```python
from build123d import *

# Parameters (mm, degrees)
SKETCH1_W                          = 70.866
SKETCH1_H                          = 25.4
SKETCH1_W_2                        = 55.372
SKETCH1_H_2                        = 19.9898
BOSS_EXTRUDE1_DEPTH                = 5.08
SKETCH7_W                          = 7.747
SKETCH7_H                          = 25.4
SKETCH7_W_2                        = 7.523824479
BOSS_EXTRUDE2_DEPTH                = 5.08
BOSS_EXTRUDE3_DEPTH                = 25.4
TAP_DRILL_FOR_6_32_TAP1_D          = 2.7051
TAP_DRILL_FOR_6_32_TAP1_DEPTH      = 10.16
TAP_DRILL_FOR_6_32_TAP1_TIP        = 0.81269403
TAP_DRILL_FOR_6_32_TAP2_AT_2_COUNT = 2
TAP_DRILL_FOR_6_32_TAP2_AT_2_PITCH = 12.7


with BuildPart() as part:
    # Sketch1 → Boss-Extrude1 (new body)
    with BuildSketch(Plane(origin=(0, 0, 0), x_dir=(1, 0, 0), z_dir=(0, 1, 0))):
        Rectangle(SKETCH1_W, SKETCH1_H)
        Rectangle(SKETCH1_W_2, SKETCH1_H_2, mode=Mode.SUBTRACT)
    extrude(amount=BOSS_EXTRUDE1_DEPTH)

    # Sketch7 → Boss-Extrude2 (add)
    with BuildSketch(Plane.XZ):
        with Locations((-31.5595, 0)):
            Rectangle(SKETCH7_W, SKETCH7_H)
        with Locations((31.671087761, 0)):
            Rectangle(SKETCH7_W_2, SKETCH7_H)
    extrude(amount=BOSS_EXTRUDE2_DEPTH)

    # Sketch8 → Boss-Extrude3 (add)
    with BuildSketch(Plane.XY.offset(12.7)):
        Polygon((35.433, 5.08), (35.433, -15.24), (39.243, -15.24), (39.243, -5.08), (39.243, 5.08), align=None)
    boss_extrude3 = extrude(amount=-BOSS_EXTRUDE3_DEPTH)

    # Mirror1: Boss-Extrude3 across plane
    add(boss_extrude3.mirror(Plane(origin=(0, 0, 0), x_dir=(0, 0, 1), z_dir=(1, 0, 0))))

    # Tap Drill for #6-32 Tap1
    with Locations(Plane(origin=(0, 5.08, 0), x_dir=(1, 0, 0), z_dir=(0, 1, 0))):
        with Locations((-32.5628, 5.0038), (-32.5628, -5.0038), (32.5628, 5.0038), (32.5628, -5.0038)):
            Hole(TAP_DRILL_FOR_6_32_TAP1_D / 2, depth=TAP_DRILL_FOR_6_32_TAP1_DEPTH)
            with Locations((0, 0, -(TAP_DRILL_FOR_6_32_TAP1_DEPTH + TAP_DRILL_FOR_6_32_TAP1_TIP / 2))):  # 118° drill point
                Cone(0, TAP_DRILL_FOR_6_32_TAP1_D / 2, TAP_DRILL_FOR_6_32_TAP1_TIP, mode=Mode.SUBTRACT)

    # Sketch10 → Tap Drill for #6-32 Tap2 (revolve, cut)
    with BuildSketch(Plane(origin=(-39.243, -8.89, -6.35), x_dir=(0, 0, 1), z_dir=(0, 1, 0))):
        Polygon((0, 0), (0, 10.97269403), (1.35255, 10.16), (1.35255, 0), align=None)
    tap_drill_for_6_32_tap2 = revolve(axis=Axis((-45.593, -8.89, -6.35), (1, 0, 0)), mode=Mode.SUBTRACT)

    # Tap Drill for #6-32 Tap2 at 2: Tap Drill for #6-32 Tap2 ×2
    with Locations(*[(0, 0, i * TAP_DRILL_FOR_6_32_TAP2_AT_2_PITCH) for i in range(1, TAP_DRILL_FOR_6_32_TAP2_AT_2_COUNT)]):
        add(tap_drill_for_6_32_tap2, mode=Mode.SUBTRACT)

    # Mirror2: Tap Drill for #6-32 Tap2 across plane
    add(tap_drill_for_6_32_tap2.mirror(Plane(origin=(0, 0, 0), x_dir=(0, 0, 1), z_dir=(1, 0, 0))), mode=Mode.SUBTRACT)

    # Mirror2 copy 1 sketch → Mirror2 copy 1 (revolve, cut)
    with BuildSketch(Plane(origin=(39.243, -8.89, 6.35), x_dir=(0, 0, 1), z_dir=(0, 1, 0))):
        Polygon((0, 0), (0, -10.97269403), (1.35255, -10.16), (1.35255, 0), align=None)
    revolve(axis=Axis((45.593, -8.89, 6.35), (1, 0, 0)), mode=Mode.SUBTRACT)


solid = part.part
```
Can you work these out from the model? Positions are in its coordinate system, mm. A direction names the side the tool comes from. Round coordinates to 2 decimals unless told otherwise and drop trailing zeros. Loops run counter-clockwise (first coordinate to the right, second up) from the corner with the lowest first, then second, coordinate; pieces in that order, holes last. Notation, with made-up numbers: M 72.5,15 L 102.5,15 A12 cw 102.5,36 Z; hole C -38.75,59.25 d1. An arc over 180 degrees is marked long. Answer as a JSON object with one key per item and string values. Group by question number.
Q1. Imagine slicing it at C-C, the plane y = 3.5. Please give me the cut outline in (x, z), then the cut area to 3 significant figures.
Q2. Will these pins go through, and if not, where does the flat tip stop? pin 1 (6 mm diameter, centred on x = -31.5, z = 2, fed in from -Y); pin 2 (2 mm diameter, centred on y = -8.89, z = -6.35, fed in from +X).
Q3. Please list where these lines run through material, in increasing order: L1, parallel to Z at x = 38.05, y = -8.89; L2, parallel to X at y = -7.5, z = 1.5; L3, parallel to Y at x = 36.95, z = -6.35.
Q4. Imagine slicing it at A-A, the plane y = -8.89. Please give me the cut outline in (x, z), then the cut area to 3 significant figures.
Q5. We'd pull the mould along X, two halves only. Please class faces 4 (the flat face through (-39.243, -5, 0)), 5 (the flat face through (-35.433, -10, 0)), 6 (the flat face through (-1, 5.08, -11)): +X half, -X half, draft (parallel to the pull), parting line (faces both ways), or undercut.
Q6. On a 3-axis mill with a long thin cutter (end or side, diameter ignored), from which of +Z, -Z, +X, -X, +Y, -Y can I reach the whole of each face in a straight line? I mean faces 1 (the flat face through (0, 1, 12.7)), 2 (the flat face through (32, -5.08, 0)), 3 (the flat face through (0, 3, -9.995)). Say none if no direction works.
Q7. Imagine slicing it at B-B, the plane x = -22. Please give me the cut outline in (y, z), then the cut area to 3 significant figures.
Findings:
{
 "1": {"outline": "M -39.24,-12.7 L 39.24,-12.7 L 39.24,12.7 L -39.24,12.7 Z; hole C -32.56,-5 d2.71; hole C -32.56,5 d2.71; hole M -27.69,-9.99 L 27.69,-9.99 L 27.69,9.99 L -27.69,9.99 Z; hole C 32.56,-5 d2.71; hole C 32.56,5 d2.71", "area": "864 mm2"},
 "2": {"pin 1": "stops at y = -5.08", "pin 2": "passes through"},
 "3": {"L1": "z = -12.7 to -7.7, -5 to 5, 7.7 to 12.7", "L2": "x = -39.24 to -35.43, 35.43 to 39.24", "L3": "y = -15.24 to -10.24, -7.54 to 5.08"},
 "4": {"outline": "M -39.24,-12.7 L -35.43,-12.7 L -35.43,-7.7 L -39.24,-7.7 Z; M -39.24,-5 L -35.43,-5 L -35.43,5 L -39.24,5 Z; M -39.24,7.7 L -35.43,7.7 L -35.43,12.7 L -39.24,12.7 Z; M 35.43,-12.7 L 39.24,-12.7 L 39.24,-7.7 L 35.43,-7.7 Z; M 35.43,-5 L 39.24,-5 L 39.24,5 L 35.43,5 Z; M 35.43,7.7 L 39.24,7.7 L 39.24,12.7 L 35.43,12.7 Z", "area": "152 mm2"},
 "5": {"face 4": "-X half", "face 5": "undercut", "face 6": "draft"},
 "6": {"face 1": "+Z, +X, -X, +Y, -Y", "face 2": "+Z, -Z, -Y", "face 3": "+Y, -Y"},
 "7": {"outline": "M 0,-12.7 L 5.08,-12.7 L 5.08,-9.99 L 0,-9.99 Z; M 0,9.99 L 5.08,9.99 L 5.08,12.7 L 0,12.7 Z", "area": "27.5 mm2"}
}
